For this review, take the finished solid that the model builds, in its own axes (mm). A direction names the side the tool comes from. Give positions to 0.01 mm unless a question says otherwise; leave off trailing zeros. Write each loop counter-clockwise with the first axis right and the second up, starting at its lowest first coordinate (ties: lowest second). Pieces come first, ordered by that corner, then holes. Notation, with made-up numbers: M -34.5,28.5 L -4.5,28.5 A26 ccw -4.5,56.5 Z; hole C 48.25,4.5 d3. An arc over 180 degrees is marked long. Use one line per item in the form item = value. Start each with the question number.
Q1. For probe 1 along Y at (x, z) = (0, 46); probe 2 along Z at (x, y) = (-9, 13.5); probe 3 along Y at (x, z) = (-13, 86.5), list the stretches that pass through material, from the lowest coordinate up. Write a range as [from, to].
Q2. Clearance check with flat-ended pins moving along their axes: pin 1 Ø6 at (x, z) = (7, 84) entering from -Y; pin 2 Ø5 at (y, z) = (11, 108) entering from -X; pin 3 Ø20 at (x, y) = (0, 0) entering from -Z; pin 4 Ø4 at (x, z) = (-11.5, 16.5) entering from -Y. State where each tip first meets the part, or that it passes through.
Q3. Mouldability with a two-part tool opening along X and no side actions: class faces 3 (the flat face through (-3, 17, 140)), 4 (the cylindrical face through (20.03, 6.31, 69.03)), 5 (the conical face through (-1.6, -7.21, 11.97)) as released by +X, released by -X, zero draft, split by the parting line, or undercut.
Q4. Consider section A-A on x = 0. Write out the cut boundary in (y, z).
Q5. Consider section C-C on z = 75. Write out the cut boundary in (x, y).
Q6. Tool access review of faces 1 (the cylindrical face through (-3.577, -16.108, 75.364)), 2 (the cylindrical face through (-5.49, -4.21, 6.42)): name each direction out of +Z, -Z, +X, -X, +Y, -Y from which nothing blocks a thin tool from reaching the whole face with its end or side.
```python
from build123d import *

# Parameters (mm, degrees)
SZKIC1_W = 140
SZKIC1_H = 21


with BuildPart() as part:
    # Szkic1 → Obr_t1 (revolve)
    with BuildSketch(Plane(origin=(0, 0, 0), x_dir=(0, 0, -1), z_dir=(1, 0, 0)), mode=Mode.PRIVATE) as obr_t1_sk:
        with Locations((-70, 10.5)):
            Rectangle(SZKIC1_W, SZKIC1_H)
    revolve(obr_t1_sk.sketch.rotate(Axis((0, 0, 0), (0, 0, 1)), 270), axis=Axis((0, 0, 0), (0, 0, 1)))

    # Szkic2 → Wyci_cie-obr_t1 (revolve, cut)
    with BuildSketch(Plane(origin=(0, 0, 0), x_dir=(0, 0, -1), z_dir=(1, 0, 0)), mode=Mode.PRIVATE) as wyci_cie_obr_t1_sk:
        Polygon((-140, 20.5), (-139.5, 21), (-140, 21), align=None)
    revolve(wyci_cie_obr_t1_sk.sketch.rotate(Axis((0, 0, 0), (0, 0, 1)), 270), axis=Axis((0, 0, 0), (0, 0, 1)), mode=Mode.SUBTRACT)

    # Szkic3 → Wyci_cie-obr_t2 (revolve, cut)
    with BuildSketch(Plane(origin=(0, 0, 0), x_dir=(0, 0, -1), z_dir=(1, 0, 0)), mode=Mode.PRIVATE) as wyci_cie_obr_t2_sk:
        Polygon((-0.5, 21), (0, 20.5), (0, 21), align=None)
    revolve(wyci_cie_obr_t2_sk.sketch.rotate(Axis((0, 0, 0), (0, 0, 1)), 270), axis=Axis((0, 0, 0), (0, 0, 1)), mode=Mode.SUBTRACT)

    # Szkic4 → Wyci_cie-obr_t3 (revolve, cut)
    with BuildSketch(Plane(origin=(0, 0, 0), x_dir=(0, 0, -1), z_dir=(1, 0, 0)), mode=Mode.PRIVATE) as wyci_cie_obr_t3_sk:
        Polygon((-13, 0), (-13, 16.5), (-11.9175, 6.9175), (-1.0825, 6.9175), (0, 8), (0, 0), align=None)
    revolve(wyci_cie_obr_t3_sk.sketch.rotate(Axis((0, 0, 0), (0, 0, 1)), 270), axis=Axis((0, 0, 0), (0, 0, 1)), mode=Mode.SUBTRACT)

    # Szkic5 → Wyci_cie-obr_t4 (revolve, cut)
    with BuildSketch(Plane(origin=(0, 0, 0), x_dir=(0, 0, -1), z_dir=(1, 0, 0)), mode=Mode.PRIVATE) as wyci_cie_obr_t4_sk:
        Polygon((-140, 0), (-140, 17), (-139.5, 16.5), (-13, 16.5), (-13, 0), align=None)
    revolve(wyci_cie_obr_t4_sk.sketch.rotate(Axis((0, 0, 13), (0, 0, 1)), 270), axis=Axis((0, 0, 13), (0, 0, 1)), mode=Mode.SUBTRACT)


solid = part.part
```
Working result:
q1.probe_1 = [-21, -16.5], [16.5, 21]
q1.probe_2 = [0, 12.97]
q1.probe_3 = [-16.49, -10.16], [10.16, 16.49]
q2.pin_1 = -20.62
q2.pin_2 = -19.2
q2.pin_3 = 0
q2.pin_4 = -18.73
q3.face_3 = zero draft
q3.face_4 = split by the parting line
q3.face_5 = undercut
q4.outline = M -21,0.5 L -20.5,0 L -8,0 L -6.92,1.08 L -6.92,11.92 L -16.5,13 L -16.5,139.5 L -17,140 L -20.5,140 L -21,139.5 Z; M 6.92,1.08 L 8,0 L 20.5,0 L 21,0.5 L 21,139.5 L 20.5,140 L 17,140 L 16.5,139.5 L 16.5,13 L 6.92,11.92 Z
q5.outline = C 0,0 d42; hole C 0,0 d33
q6.face_1 = +Z
q6.face_2 = +Z, -Z
